```python
from build123d import *

# Parameters (mm, degrees)
SKETCH1_R           = 90
BOSS_EXTRUDE1_DEPTH = 70
SKETCH3_W           = 12
SKETCH3_H           = 12
BOSS_EXTRUDE2_DEPTH = 70
FILLET1_R           = 3
SKETCH2_R           = 87
CUT_EXTRUDE3_DEPTH  = 197.859070299
SKETCH5_R           = 2.75
CUT_EXTRUDE4_DEPTH  = 197.859070299


with BuildPart() as part:
    # Sketch1 → Boss-Extrude1 (new body)
    with BuildSketch(Plane(origin=(0, 0, 0), x_dir=(1, 0, 0), z_dir=(0, 1, 0))):
        with Locations(Location((46.842609329, -26.131207683, 0), (0, 0, 270))):
            Circle(SKETCH1_R)
    extrude(amount=BOSS_EXTRUDE1_DEPTH)

    # Sketch3 → Boss-Extrude2 (add)
    with BuildSketch(Plane(origin=(0, 70, 0), x_dir=(1, 0, 0), z_dir=(0, 1, 0))):
        Polygon((139.785141997, 11.427887368), (128.372463802, 7.719683436), (132.080667734, -3.69299476), (143.49334593, 0.015209173), align=None)
        with Locations((45.842609329, 67.868792317)):
            Rectangle(SKETCH3_W, SKETCH3_H)
        Polygon((111.284253518, -102.918410355), (104.230830491, -93.210206422), (94.522626558, -100.26362945), (101.576049586, -109.971833382), align=None)
        Polygon((-6.27279694, -111.147403887), (0.780626087, -101.439199954), (-8.927577845, -94.385776927), (-15.981000873, -104.093980859), align=None)
        Polygon((-50.426161262, -1.88690386), (-39.013483066, -5.595107792), (-35.305279134, 5.817570403), (-46.717957329, 9.525774336), align=None)
    extrude(amount=-BOSS_EXTRUDE2_DEPTH)

    # Fillet1
    fillet1_edges = [part.edges().sort_by_distance(p)[0] for p in [
        (51.842609329, 35, -73.868792317),
        (39.842609329, 35, -63.59615715),
        (39.842609329, 35, -73.868792317),
        (51.842609329, 35, -63.729796095),
        (143.49334593, 35, -0.015209173),
        (139.785141997, 35, -11.427887368),
        (133.850587504, 35, 3.117912966),
        (130.015285383, 35, -8.253468525),
        (101.576049586, 35, 109.971833382),
        (111.284253518, 35, 102.918410355),
        (95.616497134, 35, 101.769213133),
        (105.246150065, 35, 94.607673928),
        (-15.981000873, 35, 104.093980859),
        (-6.27279694, 35, 111.147403887),
        (-10.02144842, 35, 95.89136061),
        (-0.234693487, 35, 102.83666746),
        (-46.717957329, 35, -9.525774336),
        (-50.426161262, 35, 1.88690386),
        (-37.075198904, 35, -6.392652197),
        (-40.656304647, 35, 5.061322703),
    ]]
    fillet(fillet1_edges, radius=FILLET1_R)

    # Sketch2 → Cut-Extrude3 (cut, through all)
    with BuildSketch(Plane(origin=(0, 70, 0), x_dir=(1, 0, 0), z_dir=(0, 1, 0))):
        with Locations(Location((46.842609329, -26.131207683, 0), (0, 0, 270))):
            Circle(SKETCH2_R)
    extrude(amount=-CUT_EXTRUDE3_DEPTH, mode=Mode.SUBTRACT)

    # Sketch5 → Cut-Extrude4 (cut, through all)
    with BuildSketch(Plane(origin=(0, 70, 0), x_dir=(1, 0, 0), z_dir=(0, 1, 0))):
        with Locations(Location((103.197332665, -101.995528399, 0), (0, 0, 270))):
            Circle(SKETCH5_R)
        with Locations(Location((-7.894080019, -103.171098904, 0), (0, 0, 270))):
            Circle(SKETCH5_R)
        with Locations(Location((-43.341248456, 2.119841769, 0), (0, 0, 270))):
            Circle(SKETCH5_R)
        with Locations(Location((45.842609329, 68.368792317, 0), (0, 0, 270))):
            Circle(SKETCH5_R)
        with Locations(Location((136.408433124, 4.021954801, 0), (0, 0, 270))):
            Circle(SKETCH5_R)
    extrude(amount=-CUT_EXTRUDE4_DEPTH, mode=Mode.SUBTRACT)


solid = part.part
```
Here's how the part is built. I have some questions about the finished solid (model axes, mm). A direction names the side the tool comes from. Give positions to 0.01 mm unless a question says otherwise; leave off trailing zeros. Write each loop counter-clockwise with the first axis right and the second up, starting at its lowest first coordinate (ties: lowest second). Pieces come first, ordered by that corner, then holes.
(1) Imagine slicing it at B-B, the plane x = 32.5. Write out the boundary of the cut face in (y, z), and give its area (3 significant figures).
Output values:
outline: (0, -62.72) - (70, -62.72) - (70, -59.68) - (0, -59.68) - close; (0, 111.94) - (70, 111.94) - (70, 114.98) - (0, 114.98) - close
area: 426 mm2
(2) Will these pins go through, and if not, where does the flat tip stop? pin 1 (9 mm diameter, centred on x = -7.89, z = 103.17, fed in from +Y); pin 2 (3.5 mm diameter, centred on y = 39, z = -69, fed in from -X); pin 3 (8 mm diameter, centred on y = 10.5, z = 16.5, fed in from -X); pin 4 (4 mm diameter, centred on x = 64, y = 17.5, fed in from -Z).
Output values:
pin 1: stops at y = 70
pin 2: stops at x = 39.84
pin 3: stops at x = -42.98
pin 4: stops at z = -62.58
(3) On a 3-axis mill with a long thin cutter (end or side, diameter ignored), from which of +Z, -Z, +X, -X, +Y, -Y can I reach the whole of each face in a straight line? I mean faces 1 (the face through (134.8, 35.49, -9.81)), 2 (the face through (106.396, 35.49, 106.47)), 3 (the face through (39.843, 35, -69)). Say none if no direction works.
Output values:
face 1: -Z, +Y, -Y
face 2: +Z, +X, +Y, -Y
face 3: -Z, -X, +Y, -Y
(4) Imagine slicing it at C-C, the plane y = 48.5. Count the separate pieces of the cut face and the enclosed holes in it, and give its area (3 significant figures).
Output values:
separate pieces: 1
enclosed holes: 6
area: 2,150 mm2
(5) If I drill on L1, parallel to X at y = 47.5, z = 27; L2, parallel to Z at x = 107.5, y = 39; L3, parallel to X at y = 23.5, z = 67, over which ranges is the centre line in solid material (lowest first)?
Output values:
L1: x = -43.15 to -40.15, 133.84 to 136.84
L2: z = -40.36 to -36.24, 88.5 to 92.62, 97.71 to 105.67
L3: x = -33.34 to -29.96, 123.65 to 127.03
(6) Imagine slicing it at A-A, the plane z = 28.5. Write out the boundary of the cut face in (x, y).
Output values:
outline: (-43.13, 0) - (-40.13, 0) - (-40.13, 70) - (-43.13, 70) - close; (133.81, 0) - (136.81, 0) - (136.81, 70) - (133.81, 70) - close
(7) Thinking about a two-plate mould opening in X: for faces 4 (the face through (51.843, 35, -69)), 5 (the face through (46, 35, -73.869)), 6 (the face through (47.15, 34.51, 116.13)), which applies, pulls with the +X half, pulls with the -X half, needs draft (parallel to the pull), parting line crosses it, or undercut?
Output values:
face 4: pulls with the +X half
face 5: needs draft
face 6: undercut
